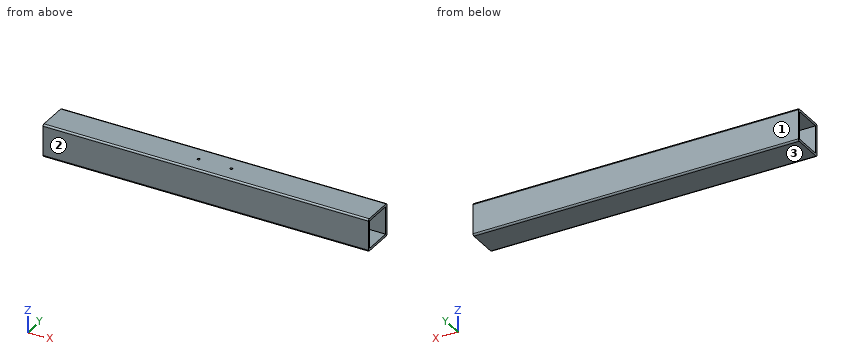
from build123d import *

# Parameters (mm, degrees)
SKETCH_W    = 34
SKETCH_H    = 34
PAD_DEPTH   = 400
SKETCH001_R = 1.65
HOLE_DEPTH  = 25
HOLE_TIPS_R = 1.65


with BuildPart() as part:
    # Sketch → Pad (new body)
    with BuildSketch(Plane.YZ):
        with BuildLine():
            Line((2, 0), (38, 0))
            ThreePointArc((38, 0), (39.414214, 0.585786), (40, 2))
            Line((40, 2), (40, 38))
            ThreePointArc((40, 38), (39.414214, 39.414214), (38, 40))
            Line((38, 40), (2, 40))
            ThreePointArc((2, 40), (0.585786, 39.414214), (0, 38))
            Line((0, 38), (0, 2))
            ThreePointArc((0, 2), (0.585786, 0.585786), (2, 0))
        make_face()
        with Locations((20, 20)):
            Rectangle(SKETCH_W, SKETCH_H, mode=Mode.SUBTRACT)
    extrude(amount=PAD_DEPTH)

    # Sketch001 (on Face5 of Pad) → Hole (cut)
    with BuildSketch(Plane(origin=(0, 0, 40), x_dir=(0, -1, 0), z_dir=(0, 0, 1))):
        with Locations((-20, 180)):
            Circle(SKETCH001_R)
        with Locations((-20, 220)):
            Circle(SKETCH001_R)
    extrude(amount=-HOLE_DEPTH, mode=Mode.SUBTRACT)

    # Hole tips → Hole tip 1 section 0
    with BuildSketch(Plane(origin=(0, 0, 15), x_dir=(0, -1, 0), z_dir=(0, 0, 1)), mode=Mode.PRIVATE) as hole_tip_1_s0:
        with Locations((-20, 180)):
            Circle(HOLE_TIPS_R)
    loft([hole_tip_1_s0.sketch, Vertex(180, 20, 14.00858)], mode=Mode.SUBTRACT)

    # Hole tips → Hole tip 2 section 0
    with BuildSketch(Plane(origin=(0, 0, 15), x_dir=(0, -1, 0), z_dir=(0, 0, 1)), mode=Mode.PRIVATE) as hole_tip_2_s0:
        with Locations((-20, 220)):
            Circle(HOLE_TIPS_R)
    loft([hole_tip_2_s0.sketch, Vertex(220, 20, 14.00858)], mode=Mode.SUBTRACT)


solid = part.part
Can you work these out from the model? Positions are in its coordinate system, mm. Face numbers are marked on the shaded views. Give positions to 0.01 mm unless a question says otherwise; leave off trailing zeros. Loops run counter-clockwise (first coordinate to the right, second up) from the corner with the lowest first, then second, coordinate; pieces in that order, holes last. Notation, with made-up numbers: (62.5, -11.5) - (86.5, -11.5) arc R22 ccw to (86.5, 3.5) - close; hole circle Ø9 at (80.5, 30.25). An arc over 180 degrees is marked (long way). Answer as a JSON object with one key per item and string values.
Q1. Imagine slicing it at C-C on x = 135. Write out the boundary of the cut face in (y, z), plus the area to 3 significant figures.
Geometry says:
{"outline": "(0, 2) arc R2 ccw to (2, 0) - (38, 0) arc R2 ccw to (40, 2) - (40, 38) arc R2 ccw to (38, 40) - (2, 40) arc R2 ccw to (0, 38) - close; hole (3, 3) - (37, 3) - (37, 37) - (3, 37) - close", "area": "441 mm²"}
Q2. Will this pin go through, and if not, where does the flat tip stop? P1, Ø2, axis at x = 220, y = 20, coming from the +Z side.
Geometry says:
{"P1": "z = 3"}
Q3. If we mould it in two halves opening along Y, with no side actions, what happens to the marked faces 1, 2 and 3? For each: pulls with the +Y half, pulls with the -Y half, needs draft (parallel to the pull), parting line crosses it, or undercut.
Geometry says:
{"face 1": "pulls with the +Y half", "face 2": "pulls with the -Y half", "face 3": "needs draft"}
Q4. If I drill on L1, parallel to X at y = 20, z = 38.3; L2, parallel to Y at x = 326, z = 3.5, over which ranges is the centre line in solid material (lowest first)?
Geometry says:
{"L1": "0 to 178.35, 181.65 to 218.35, 221.65 to 400", "L2": "0 to 3, 37 to 40"}
Q5. Imagine slicing it at A-A on y = 12.5. Write out the boundary of the cut face in (x, z).
Geometry says:
{"outline": "(0, 0) - (400, 0) - (400, 3) - (0, 3) - close; (0, 37) - (400, 37) - (400, 40) - (0, 40) - close"}
